Here's how the part is built. I have some questions about the finished solid (model axes, mm). Face numbers are marked on the shaded views. A direction names the side the tool comes from. Coordinates: 2 decimals unless noted, no trailing zeros. Write each loop counter-clockwise with the first axis right and the second up, starting at its lowest first coordinate (ties: lowest second). Pieces come first, ordered by that corner, then holes.
Item 1: For the marked faces 4 and 5, which set-ups out of +Z, -Z, +X, -X, +Y, -Y let a thin tool reach every point of the face, with its end or its side?
Item 2: If we mould it in two halves opening along X, with no side actions, what happens to the marked faces 1, 2 and 3? For each: pulls with the +X half, pulls with the -X half, needs draft (parallel to the pull), parting line crosses it, or undercut.
Item 3: I want a section at A-A (x = 0). Please give me the cut outline in (y, z), and give its area (3 significant figures).
Item 4: I want a section at C-C (x = -20.5). Please give me the cut outline in (y, z), and give its area (3 significant figures).
Item 5: Please list where these lines run through material, in increasing order: line 1 (X direction, y = 39, z = 13); line 2 (X direction, y = 35.5, z = 12); line 3 (Y direction, x = -20.5, z = 1.5).
Item 6: I want a section at D-D (z = 4.75). Please give me the cut outline in (x, y).
Item 7: I want a section at B-B (y = 39). Please give me the cut outline in (x, z).
Item 8: I'm going to push flat-ended pins straight in: P1, Ø1.5, axis at y = 1, z = 10.5, coming from the +X side; P2, Ø6, axis at x = -25.5, z = 6, coming from the +Y side; P3, Ø7, axis at x = -39, y = 0, coming from the +Z side. Where does each tip first touch, or does it pass through?
from build123d import *

# Parameters (mm, degrees)
SKETCH_1_R               = 44
SKETCH_1_R_2             = 34
EXTRUDE_1_DEPTH          = 15
SKETCH_2_R               = 4.5
CUT_EXTRUDE_1_DEPTH      = 6
SKETCH_3_R               = 2.5
CUT_EXTRUDE_2_DEPTH      = 11
PATTERN_CIRCULAR_1_COUNT = 4


with BuildPart() as part:
    # 草图1 → 凸台-拉伸1 (new body)
    with BuildSketch(Plane.XY):
        Circle(SKETCH_1_R)
        Circle(SKETCH_1_R_2, mode=Mode.SUBTRACT)
    extrude(amount=EXTRUDE_1_DEPTH)

    # 草图2 → 切除-拉伸1 (cut)
    with BuildSketch(Plane.XY.offset(15)):
        with Locations((39, 0)):
            Circle(SKETCH_2_R)
    cut_extrude_1 = extrude(amount=-CUT_EXTRUDE_1_DEPTH, mode=Mode.SUBTRACT)

    # 草图3 → 切除-拉伸2 (cut)
    with BuildSketch(Plane.XY.offset(9)):
        with Locations((39, 0)):
            Circle(SKETCH_3_R)
    cut_extrude_2 = extrude(amount=-CUT_EXTRUDE_2_DEPTH, mode=Mode.SUBTRACT)

    # 阵列(圆周)1: 切除-拉伸1, 切除-拉伸2 ×4 about axis
    pattern_circular_1_axis = Axis((0, 0, 0), (0, 0, 1))
    for i in range(1, PATTERN_CIRCULAR_1_COUNT):
        add(cut_extrude_1.rotate(pattern_circular_1_axis, i * 360 / PATTERN_CIRCULAR_1_COUNT), mode=Mode.SUBTRACT)
        add(cut_extrude_2.rotate(pattern_circular_1_axis, i * 360 / PATTERN_CIRCULAR_1_COUNT), mode=Mode.SUBTRACT)


solid = part.part
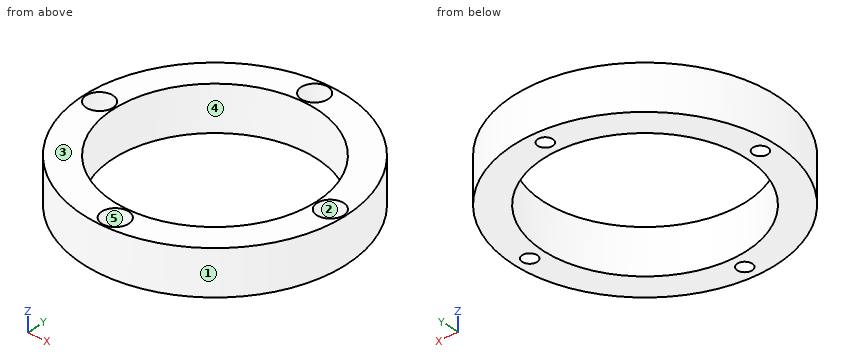
Answer:
1. face 4: +Z, -Z
1. face 5: +Z
2. face 1: parting line crosses it
2. face 2: undercut
2. face 3: needs draft
3. outline: (-44, 0) - (-41.5, 0) - (-41.5, 9) - (-43.5, 9) - (-43.5, 15) - (-44, 15) - close; (-36.5, 0) - (-34, 0) - (-34, 15) - (-34.5, 15) - (-34.5, 9) - (-36.5, 9) - close; (34, 0) - (36.5, 0) - (36.5, 9) - (34.5, 9) - (34.5, 15) - (34, 15) - close; (41.5, 0) - (44, 0) - (44, 15) - (43.5, 15) - (43.5, 9) - (41.5, 9) - close
3. area: 102 mm2
4. outline: (-38.93, 0) - (-27.12, 0) - (-27.12, 15) - (-38.93, 15) - close; (27.12, 0) - (38.93, 0) - (38.93, 15) - (27.12, 15) - close
4. area: 354 mm2
5. line 1: x = -20.37 to -4.5, 4.5 to 20.37
5. line 2: x = -26 to -2.83, 2.83 to 26
5. line 3: y = -38.93 to -27.12, 27.12 to 38.93
6. outline: circle Ø88 at (0, 0); hole circle Ø5 at (-39, 0); hole circle Ø68 at (0, 0); hole circle Ø5 at (0, -39); hole circle Ø5 at (0, 39); hole circle Ø5 at (39, 0)
7. outline: (-20.37, 0) - (-2.5, 0) - (-2.5, 9) - (-4.5, 9) - (-4.5, 15) - (-20.37, 15) - close; (2.5, 0) - (20.37, 0) - (20.37, 15) - (4.5, 15) - (4.5, 9) - (2.5, 9) - close
8. P1: stops at x = 44
8. P2: stops at y = 37.81
8. P3: stops at z = 9
